CAD build for the part. Positions are in the model's coordinates, mm. Round coordinates to 2 decimals unless told otherwise and drop trailing zeros. Order: outer loops, then holes, each group sorted by start corner. A loop starts at its lowest first (then second) coordinate and runs counter-clockwise, first axis right, second up. Notation, with made-up numbers: (2, 44.5) - (45, 44.5) arc R12 ccw to (45, 64.5) - close; hole circle Ø7 at (77.25, 24). An arc over 180 degrees is marked (long way). Use one line per item in the form item = value. Start each with the question number.
from build123d import *

# Parameters (mm, degrees)
BOSS_EXTRUDE1_DEPTH            = 6.35
SKETCH3_W                      = 6.35
SKETCH3_H                      = 31.75
SKETCH3_H_2                    = 29.028571429
CUT_EXTRUDE1_DEPTH             = 419.66682159
SKETCH4_R                      = 1.5
CUT_EXTRUDE2_DEPTH             = 6.35
SKETCH5_W                      = 6.35
SKETCH5_H                      = 44.45
SKETCH5_W_2                    = 59.592307692
SKETCH5_H_2                    = 6.35
CUT_EXTRUDE3_DEPTH             = 6.35
SKETCH6_W                      = 6.35
SKETCH6_H                      = 222.25
BOSS_EXTRUDE2_DEPTH            = 6.35
SKETCH7_W                      = 774.7
SKETCH7_H                      = 14.696452311
CUT_EXTRUDE4_DEPTH             = 6.35
SKETCH8_R                      = 1.190625
HOLES_FOR_PLASTIC_SCREWS_DEPTH = 10


with BuildPart() as part:
    # Sketch1 → Boss-Extrude1 (new body)
    with BuildSketch(Plane(origin=(0, 0, 0), x_dir=(0, 0, -1), z_dir=(1, 0, 0))):
        Polygon((-387.35, 152.4), (-387.35, 107.95), (-381, 107.95), (-381, 63.5), (-387.35, 63.5), (-387.35, 19.05), (-381, 19.05), (-381, -25.4), (-387.35, -25.4), (-387.35, -69.85), (-381, -69.85), (-381, -114.3), (-387.35, -114.3), (-387.35, -152.4), (-327.757692308, -152.4), (-327.757692308, -158.75), (-268.165384615, -158.75), (-268.165384615, -152.4), (-208.573076923, -152.4), (-208.573076923, -158.75), (-148.980769231, -158.75), (-148.980769231, -152.4), (-89.388461538, -152.4), (-89.388461538, -158.75), (-29.796153846, -158.75), (-29.796153846, -152.4), (29.796153846, -152.4), (29.796153846, -158.75), (89.388461538, -158.75), (89.388461538, -152.4), (148.980769231, -152.4), (148.980769231, -158.75), (208.573076923, -158.75), (208.573076923, -152.4), (268.165384615, -152.4), (268.165384615, -158.75), (327.757692308, -158.75), (327.757692308, -152.4), (387.35, -152.4), (387.35, -114.3), (381, -114.3), (381, -69.85), (387.35, -69.85), (387.35, -25.4), (381, -25.4), (381, 19.05), (387.35, 19.05), (387.35, 63.5), (381, 63.5), (381, 107.95), (387.35, 107.95), (387.35, 152.4), align=None)
    extrude(amount=BOSS_EXTRUDE1_DEPTH)

    # Sketch3 → Cut-Extrude1 (cut, through all)
    with BuildSketch(Plane(origin=(6.35, 0, 0), x_dir=(0, 0, -1), z_dir=(1, 0, 0))):
        with Locations((-120.648769685, -104.775)):
            Rectangle(SKETCH3_W, SKETCH3_H)
        with Locations((-120.648769685, -41.275)):
            Rectangle(SKETCH3_W, SKETCH3_H)
        with Locations((-120.648769685, 22.225)):
            Rectangle(SKETCH3_W, SKETCH3_H)
        with Locations((-120.648769685, 85.725)):
            Rectangle(SKETCH3_W, SKETCH3_H)
        with Locations((-133.351230315, 61.685714285)):
            Rectangle(SKETCH3_W, SKETCH3_H_2)
        with Locations((-133.351230315, 3.628571428)):
            Rectangle(SKETCH3_W, SKETCH3_H_2)
        with Locations((-133.351230315, -54.428571428)):
            Rectangle(SKETCH3_W, SKETCH3_H_2)
        with Locations((-133.351230315, -112.485714286)):
            Rectangle(SKETCH3_W, SKETCH3_H_2)
        with Locations((133.351230315, 85.725)):
            Rectangle(SKETCH3_W, SKETCH3_H)
        with Locations((120.648769685, 61.685714285)):
            Rectangle(SKETCH3_W, SKETCH3_H_2)
        with Locations((133.351230315, 22.225)):
            Rectangle(SKETCH3_W, SKETCH3_H)
        with Locations((120.648769685, 3.628571428)):
            Rectangle(SKETCH3_W, SKETCH3_H_2)
        with Locations((133.351230315, -41.275)):
            Rectangle(SKETCH3_W, SKETCH3_H)
        with Locations((120.648769685, -54.428571428)):
            Rectangle(SKETCH3_W, SKETCH3_H_2)
        with Locations((133.351230315, -104.775)):
            Rectangle(SKETCH3_W, SKETCH3_H)
        with Locations((120.648769685, -112.485714286)):
            Rectangle(SKETCH3_W, SKETCH3_H_2)
    extrude(amount=-CUT_EXTRUDE1_DEPTH, mode=Mode.SUBTRACT)

    # Sketch4 → Cut-Extrude2 (cut)
    with BuildSketch(Plane(origin=(6.35, 0, 0), x_dir=(0, 0, -1), z_dir=(1, 0, 0))):
        with Locations((-368.3, 137.4)):
            Circle(SKETCH4_R)
        with Locations((-368.3, 121.65)):
            Circle(SKETCH4_R)
        with Locations((368.3, 137.4)):
            Circle(SKETCH4_R)
        with Locations((368.3, 121.65)):
            Circle(SKETCH4_R)
    extrude(amount=-CUT_EXTRUDE2_DEPTH, mode=Mode.SUBTRACT)

    # Sketch5 → Cut-Extrude3 (cut)
    with BuildSketch(Plane(origin=(6.35, 0, 0), x_dir=(0, 0, -1), z_dir=(1, 0, 0))):
        with Locations((-384.175, 41.275)):
            Rectangle(SKETCH5_W, SKETCH5_H)
        with Locations((-384.175, -47.625)):
            Rectangle(SKETCH5_W, SKETCH5_H)
        with Locations((-178.776923077, -155.575)):
            Rectangle(SKETCH5_W_2, SKETCH5_H_2)
        with Locations((-59.592307692, -155.575)):
            Rectangle(SKETCH5_W_2, SKETCH5_H_2)
        with Locations((59.592307692, -155.575)):
            Rectangle(SKETCH5_W_2, SKETCH5_H_2)
        with Locations((178.776923077, -155.575)):
            Rectangle(SKETCH5_W_2, SKETCH5_H_2)
        with Locations((384.175, -47.625)):
            Rectangle(SKETCH5_W, SKETCH5_H)
        with Locations((384.175, 41.275)):
            Rectangle(SKETCH5_W, SKETCH5_H)
    extrude(amount=-CUT_EXTRUDE3_DEPTH, mode=Mode.SUBTRACT)

    # Sketch6 → Boss-Extrude2 (add)
    with BuildSketch(Plane(origin=(6.35, 0, 0), x_dir=(0, 0, -1), z_dir=(1, 0, 0))):
        with Locations((-384.175, -3.175)):
            Rectangle(SKETCH6_W, SKETCH6_H)
        with Locations((384.175, -3.175)):
            Rectangle(SKETCH6_W, SKETCH6_H)
    extrude(amount=-BOSS_EXTRUDE2_DEPTH)

    # Sketch7 → Cut-Extrude4 (cut)
    with BuildSketch(Plane(origin=(6.35, 0, 0), x_dir=(0, 0, -1), z_dir=(1, 0, 0))):
        with Locations((0, -159.748226155)):
            Rectangle(SKETCH7_W, SKETCH7_H)
    extrude(amount=-CUT_EXTRUDE4_DEPTH, mode=Mode.SUBTRACT)

    # Sketch8 → Holes for plastic screws (cut)
    with BuildSketch(Plane(origin=(6.35, 0, 0), x_dir=(0, 0, -1), z_dir=(1, 0, 0))):
        with Locations((384.175, 101.6)):
            Circle(SKETCH8_R)
        with Locations((384.175, 0)):
            Circle(SKETCH8_R)
        with Locations((384.175, -101.6)):
            Circle(SKETCH8_R)
        with Locations((-384.175, -101.6)):
            Circle(SKETCH8_R)
        with Locations((-384.175, 0)):
            Circle(SKETCH8_R)
        with Locations((-384.175, 101.6)):
            Circle(SKETCH8_R)
    extrude(amount=-HOLES_FOR_PLASTIC_SCREWS_DEPTH, mode=Mode.SUBTRACT)


solid = part.part
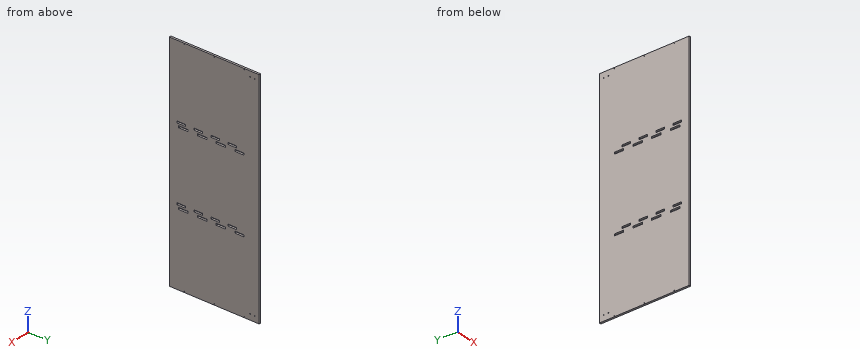
(1) Flat gauge pin, fed straight in: P1, Ø1.9, axis at y = 101.6, z = -384.175, coming from the -X side. Where does the tip first touch, or does it go through?
(2) Slice it at A-A (y = 60). Give the cut face in (x, z).
(3) Wall check: line 1 (Z direction, x = 6.25, y = -107.5); line 2 (Z direction, x = 6.25, y = 88); line 3 (Z direction, x = 0.75, y = -61.5). Give the ranges that are in metal, low to high. Write a range as [from, to].
Results list:
q1.P1 = through
q2.outline = (0, -387.35) - (6.35, -387.35) - (6.35, -123.82) - (0, -123.82) - close; (0, -117.47) - (6.35, -117.47) - (6.35, 130.18) - (0, 130.18) - close; (0, 136.53) - (6.35, 136.53) - (6.35, 387.35) - (0, 387.35) - close
q3.line_1 = [-387.35, -136.53], [-130.18, -123.82], [-117.47, 117.47], [123.82, 130.18], [136.53, 387.35]
q3.line_2 = [-387.35, -136.53], [-130.18, 117.47], [123.82, 387.35]
q3.line_3 = [-387.35, -123.82], [-117.47, 130.18], [136.53, 387.35]
